Geometry: see drawing. Coordinates: mm, zero at the bounding-box minimum. A direction names the side the tool comes from. Round coordinates to 2 decimals unless told otherwise and drop trailing zeros. Loops run counter-clockwise (first coordinate to the right, second up) from the corner with the lowest first, then second, coordinate; pieces in that order, holes last. Notation, with made-up numbers: (63, 89) -> (113, 89) arc R8 ccw to (113, 93) -> close; hole circle Ø7 at (7, 56). An arc over 180 degrees is marked (long way). Write item = value, one per line.
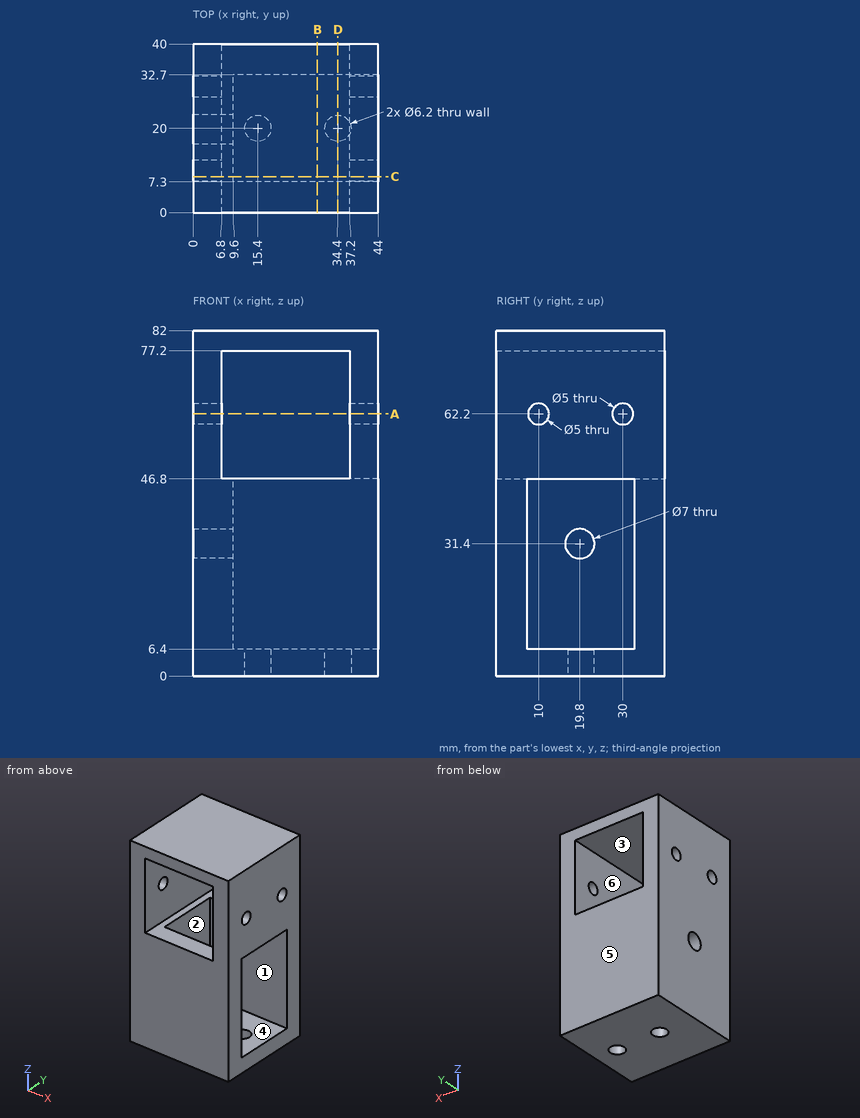
1. Contact query for a flat-ended pin moving along its axis: pin 1 Ø12 at (x, z) = (15, 25) entering from -Y. Output: stop coordinate, or through.
Evaluation:
pin_1 = 0
2. Section query B-B (x = 29.5). Return the cut outline in (y, z), then the cut area to 3 significant figures.
Evaluation:
outline = (0, 0) -> (40, 0) -> (40, 46.8) -> (32.7, 46.8) -> (32.7, 6.4) -> (7.3, 6.4) -> (7.3, 46.8) -> (0, 46.8) -> close; (0, 77.2) -> (40, 77.2) -> (40, 82) -> (0, 82) -> close
area = 1,040 mm²
3. Line query: probe 1 along Y at (x, z) = (40.75, 62.2); probe 2 along Z at (x, y) = (10.5, 14); probe 3 along Z at (x, y) = (9, 12.5). Output: solid intervals per line, ascending. Write a range as from..to.
Evaluation:
probe_1 = 0..7.5, 12.5..27.5, 32.5..40
probe_2 = 0..6.4, 77.2..82
probe_3 = 0..46.8, 77.2..82
4. Mould query, pull axis X, two halves, no side actions, for the marked faces 1, 2 and 3. Classes: released by +X, released by -X, zero draft, split by the parting line, or undercut.
Evaluation:
face_1 = zero draft
face_2 = released by +X
face_3 = undercut
5. Section query C-C (y = 8.5). Return the cut outline in (x, z).
Evaluation:
outline = (0, 0) -> (44, 0) -> (44, 6.4) -> (9.6, 6.4) -> (9.6, 46.8) -> (6.8, 46.8) -> (6.8, 60.2) -> (0, 60.2) -> close; (0, 64.2) -> (6.8, 64.2) -> (6.8, 77.2) -> (37.2, 77.2) -> (37.2, 64.2) -> (44, 64.2) -> (44, 82) -> (0, 82) -> close; (37.2, 46.8) -> (44, 46.8) -> (44, 60.2) -> (37.2, 60.2) -> close
6. Section query A-A (z = 62.2). Return the cut outline in (x, y).
Evaluation:
outline = (0, 0) -> (6.8, 0) -> (6.8, 7.5) -> (0, 7.5) -> close; (0, 12.5) -> (6.8, 12.5) -> (6.8, 27.5) -> (0, 27.5) -> close; (0, 32.5) -> (6.8, 32.5) -> (6.8, 40) -> (0, 40) -> close; (37.2, 0) -> (44, 0) -> (44, 7.5) -> (37.2, 7.5) -> close; (37.2, 12.5) -> (44, 12.5) -> (44, 27.5) -> (37.2, 27.5) -> close; (37.2, 32.5) -> (44, 32.5) -> (44, 40) -> (37.2, 40) -> close
7. Section query D-D (x = 34.4). Return the cut outline in (y, z), then the cut area to 3 significant figures.
Evaluation:
outline = (0, 0) -> (16.9, 0) -> (16.9, 6.4) -> (7.3, 6.4) -> (7.3, 46.8) -> (0, 46.8) -> close; (0, 77.2) -> (40, 77.2) -> (40, 82) -> (0, 82) -> close; (23.1, 0) -> (40, 0) -> (40, 46.8) -> (32.7, 46.8) -> (32.7, 6.4) -> (23.1, 6.4) -> close
area = 998 mm²
8. Set-up query: the marked faces 4, 5 and 6. Return all of +Z, -Z, +X, -X, +Y, -Y with unobstructed straight access to the full face (end or side cutting, diameter ignored); none if empty.
Evaluation:
face_4 = +X
face_5 = +Z, -Z, +X, -X, +Y
face_6 = +Y, -Y
